Input: dimensioned drawing with shaded views. Units: mm. Origin: part minimum x, y, z. Coordinates: 2 decimals unless noted, no trailing zeros. Order: outer loops, then holes, each group sorted by start corner. A loop starts at its lowest first (then second) coordinate and runs counter-clockwise, first axis right, second up. Notation, with made-up numbers: M -34.75,-29 L -13.75,-29 A20 ccw -13.75,-8 Z; hole C 63.5,-28 d6. An arc over 180 degrees is marked long. Use CSV: the item, a comma, the result in double quotes. Start each with the question number.
1. First-contact query: P1, Ø1, axis at x = 47, y = 0.5, coming from the -Z side; P2, Ø1, axis at x = 22.5, y = 0.5, coming from the -Z side. Flat tips, straight axial feed; report the tip coordinate or a pass-through.
2. Section query A-A on z = 20. Return the cut outline in (x, y), and give its area (3 significant figures).
3. Material intervals for line 1 (X direction, y = 0.9, z = 20); line 2 (X direction, y = 1.45, z = 18.5); line 3 (Z direction, x = 13.5, y = 0.75), sorted ascending.
4. Section query C-C on x = 50. Return the cut outline in (y, z).
5. Section query B-B on y = 1.3. Return the cut outline in (x, z), and give its area (3 significant figures).
6. Section query D-D on z = 7.5. Return the cut outline in (x, y), and give its area (3 significant figures).
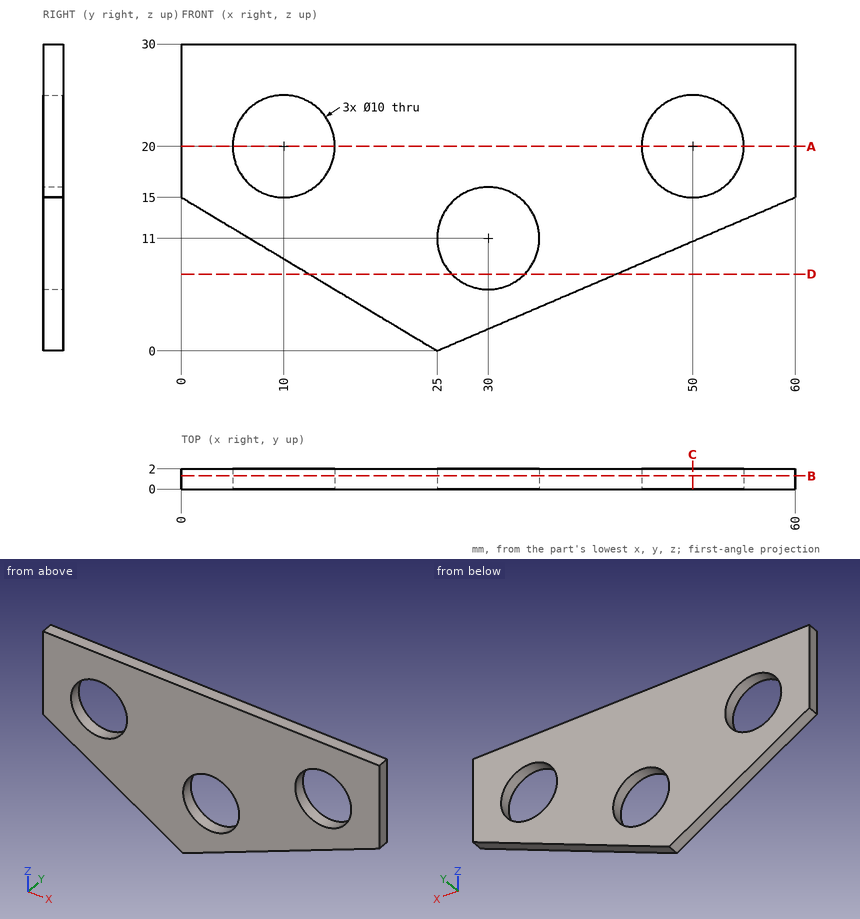
Results list:
1,P1,"stops at z = 9.21"
1,P2,"stops at z = 1.2"
2,outline,"M 0,0 L 5,0 L 5,2 L 0,2 Z; M 15,0 L 45,0 L 45,2 L 15,2 Z; M 55,0 L 60,0 L 60,2 L 55,2 Z"
2,area,"80.0 mm²"
3,line 1,"x = 0 to 5, 15 to 45, 55 to 60"
3,line 2,"x = 0 to 5.23, 14.77 to 45.23, 54.77 to 60"
3,line 3,"z = 6.9 to 16.43, 23.57 to 30"
4,outline,"M 0,10.71 L 2,10.71 L 2,15 L 0,15 Z; M 0,25 L 2,25 L 2,30 L 0,30 Z"
5,outline,"M 0,15 L 25,0 L 60,15 L 60,30 L 0,30 Z; hole C 10,20 d10; hole C 30,11 d10; hole C 50,20 d10"
5,area,"1,110 mm²"
6,outline,"M 12.5,0 L 26.43,0 L 26.43,2 L 12.5,2 Z; M 33.57,0 L 42.5,0 L 42.5,2 L 33.57,2 Z"
6,area,"45.7 mm²"
